Design review of the part built by this model. Coordinates are the model's own, in mm. A direction names the side the tool comes from. Give positions to 0.01 mm unless a question says otherwise; leave off trailing zeros. Write each loop counter-clockwise with the first axis right and the second up, starting at its lowest first coordinate (ties: lowest second). Pieces come first, ordered by that corner, then holes.
```python
from build123d import *

# Parameters (mm, degrees)
BOSS_EXTRUDE1_DEPTH = 152.4
FILLET1_R           = 3.175
SKETCH2_R           = 3.175
CUT_EXTRUDE2_DEPTH  = 152.4
CHAMFER1_SIZE       = 2.54
CHAMFER2_SIZE       = 2.54
SKETCH3_R           = 3.175
CUT_EXTRUDE3_DEPTH  = 152.4
CUT_EXTRUDE4_DEPTH  = 152.4


with BuildPart() as part:
    # Sketch1 → Boss-Extrude1 (new body)
    with BuildSketch(Plane(origin=(0, 0, 0), x_dir=(0, 0, -1), z_dir=(1, 0, 0))):
        Polygon((19.05, -19.05), (-19.05, -19.05), (-19.05, -12.7), (12.7, -12.7), (12.7, 19.05), (19.05, 19.05), align=None)
    extrude(amount=BOSS_EXTRUDE1_DEPTH)

    # Fillet1
    fillet1_edges = [part.edges().sort_by_distance(p)[0] for p in [
        (76.2, -12.7, -12.7),
    ]]
    fillet(fillet1_edges, radius=FILLET1_R)

    # Sketch2 → Cut-Extrude2 (cut)
    with BuildSketch(Plane(origin=(0, 0, -19.05), x_dir=(-1, 0, 0), z_dir=(0, 0, -1))):
        with Locations((-104.775, 6.35)):
            Circle(SKETCH2_R)
        with Locations((-76.2, 6.35)):
            Circle(SKETCH2_R)
        with Locations((-47.625, 6.35)):
            Circle(SKETCH2_R)
    extrude(amount=-CUT_EXTRUDE2_DEPTH, mode=Mode.SUBTRACT)

    # Chamfer1
    chamfer1_edges = [part.edges().sort_by_distance(p)[0] for p in [
        (50.8, 6.35, -12.7),
    ]]
    chamfer(chamfer1_edges, length=CHAMFER1_SIZE)

    # Chamfer2
    chamfer2_edges = [part.edges().sort_by_distance(p)[0] for p in [
        (107.95, 6.35, -12.7),
        (79.375, 6.35, -12.7),
    ]]
    chamfer(chamfer2_edges, length=CHAMFER2_SIZE)

    # Sketch3 → Cut-Extrude3 (cut)
    with BuildSketch(Plane(origin=(0, -12.7, 0), x_dir=(1, 0, 0), z_dir=(0, 1, 0))):
        with Locations(Location((19.05, -6.35, 0), (0, 0, 270))):
            Circle(SKETCH3_R)
        with Locations(Location((57.15, -6.35, 0), (0, 0, 270))):
            Circle(SKETCH3_R)
        with Locations(Location((95.25, -6.35, 0), (0, 0, 270))):
            Circle(SKETCH3_R)
        with Locations(Location((133.35, -6.35, 0), (0, 0, 270))):
            Circle(SKETCH3_R)
    extrude(amount=-CUT_EXTRUDE3_DEPTH, mode=Mode.SUBTRACT)

    # Sketch4 → Cut-Extrude4 (cut)
    with BuildSketch(Plane(origin=(0, 0, -19.05), x_dir=(-1, 0, 0), z_dir=(0, 0, -1))):
        Polygon((-152.4, -19.05), (-114.3, 19.05), (-152.4, 19.05), align=None)
        Polygon((0, -19.05), (-38.1, 19.05), (0, 19.05), align=None)
    extrude(amount=-CUT_EXTRUDE4_DEPTH, mode=Mode.SUBTRACT)


solid = part.part
```
(1) Consider section D-D, the plane x = 76.2. Give the boundary of the cut face in (y, z) (3 decimals), then the cut area to 3 significant figures.
Resolved:
outline: (-19.05, -19.05) - (3.175, -19.05) - (3.175, -15.24) - (0.635, -12.7) - (-9.525, -12.7) arc R3.175 cw to (-12.7, -9.525) - (-12.7, 19.05) - (-19.05, 19.05) - close; (9.525, -19.05) - (19.05, -19.05) - (19.05, -12.7) - (12.065, -12.7) - (9.525, -15.24) - close
area: 399 mm2
(2) Consider section A-A, the plane x = 133.35. Give the boundary of the cut face in (y, z) (3 decimals), then the cut area to 3 significant figures.
Resolved:
outline: (-19.05, -19.05) - (0, -19.05) - (0, -12.7) - (-9.525, -12.7) arc R3.175 cw to (-12.7, -9.525) - (-12.7, 3.175) - (-19.05, 3.175) - close; (-19.05, 9.525) - (-12.7, 9.525) - (-12.7, 19.05) - (-19.05, 19.05) - close
area: 284 mm2
(3) Tool access review of faces 1 (the face through (75, -2, -12.7)), 2 (the face through (107.947, 6.49, -17.172)): name each direction out of +Z, -Z, +X, -X, +Y, -Y from which nothing blocks a thin tool from reaching the whole face with its end or side.
Resolved:
face 1: +Z, +X, -X, +Y
face 2: +Z, -Z
(4) Consider section C-C, the plane z = 6.35. Give the boundary of the cut face in (x, y) (3 decimals), then the cut area to 3 significant figures.
Resolved:
outline: (0, -19.05) - (15.875, -19.05) - (15.875, -12.7) - (6.35, -12.7) - close; (22.225, -19.05) - (53.975, -19.05) - (53.975, -12.7) - (22.225, -12.7) - close; (60.325, -19.05) - (92.075, -19.05) - (92.075, -12.7) - (60.325, -12.7) - close; (98.425, -19.05) - (130.175, -19.05) - (130.175, -12.7) - (98.425, -12.7) - close; (136.525, -19.05) - (152.4, -19.05) - (146.05, -12.7) - (136.525, -12.7) - close
area: 766 mm2
(5) Consider section B-B, the plane y = 6.35. Give the boundary of the cut face in (x, z) (3 decimals), then the cut area to 3 significant figures.
Resolved:
outline: (25.4, -19.05) - (44.45, -19.05) - (44.45, -15.24) - (41.91, -12.7) - (25.4, -12.7) - close; (50.8, -19.05) - (73.025, -19.05) - (73.025, -15.24) - (70.485, -12.7) - (53.34, -12.7) - (50.8, -15.24) - close; (79.375, -19.05) - (101.6, -19.05) - (101.6, -15.24) - (99.06, -12.7) - (81.915, -12.7) - (79.375, -15.24) - close; (107.95, -19.05) - (127, -19.05) - (127, -12.7) - (110.49, -12.7) - (107.95, -15.24) - close
area: 505 mm2
(6) Mouldability with a two-part tool opening along Y and no side actions: class faces 3 (the face through (75, -16, 19.05)), 4 (the face through (75, -19.05, 0)), 5 (the face through (101.73, 5.09, -15.12)) as pulls with the +Y half, pulls with the -Y half, needs draft (parallel to the pull), parting line crosses it, or undercut.
Resolved:
face 3: needs draft
face 4: pulls with the -Y half
face 5: undercut
(7) To check wall thickness, follow L1, parallel to Z at x = 19, y = -17; L2, parallel to X at y = -13.75, z = 6.35 (3 decimals); L3, parallel to Y at x = 76.2, z = -16.2 (3 decimals). State the ranges of each line that lie inside material, in increasing order.
Resolved:
L1: z = -19.05 to 3.18, 9.52 to 19.05
L2: x = 5.3 to 15.875, 22.225 to 53.975, 60.325 to 92.075, 98.425 to 130.175, 136.525 to 147.1
L3: y = -19.05 to 3.175, 9.525 to 19.05
(8) Clearance check with flat-ended pins moving along their axes: P1, Ø8.5, axis at x = 63.5, y = -0.5, coming from the +Z side; P2, Ø6, axis at x = 98, z = 3, coming from the +Y side; P3, Ø10, axis at x = 76.2, y = 6.35, coming from the +Z side (3 decimals). State where each tip first meets the part, or that it passes through.
Resolved:
P1: stops at z = -12.7
P2: stops at y = -12.7
P3: stops at z = -13.415
